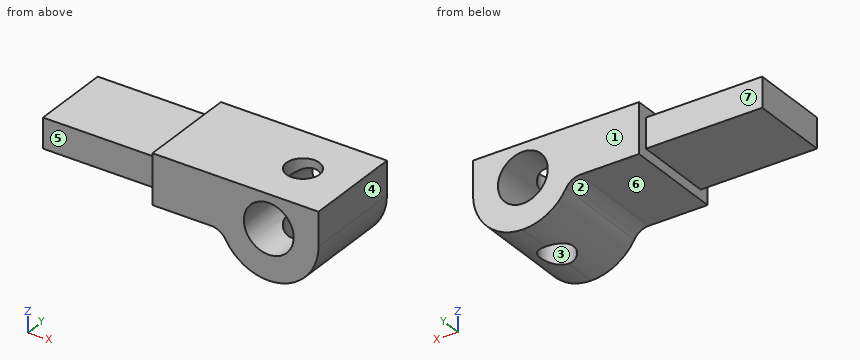
from build123d import *

# Parameters (mm, degrees)
BOSS_EXTRUDE1_DEPTH      = 38.1
BOSS_EXTRUDE1_DEPTH_BACK = 38.1
CUT_EXTRUDE1_DEPTH       = 84.279469259
CUT_EXTRUDE1_DEPTH_BACK  = 84.279469259
SKETCH4_R                = 12.7
SKETCH5_W                = 22.86
SKETCH5_H                = 60.96
BOSS_EXTRUDE2_DEPTH      = 88.9
SKETCH6_R                = 19.05
CUT_EXTRUDE2_DEPTH       = 175.596134043


with BuildPart() as part:
    # Sketch2 → Boss-Extrude1 (new, two sides: drawn at the far end of the back side and taken through both)
    with BuildSketch(Plane(origin=(0, 0, 0), x_dir=(1, 0, 0), z_dir=(0, 1, 0)).offset(-BOSS_EXTRUDE1_DEPTH_BACK)):
        with BuildLine():
            Line((-63.5, 12.7), (-63.5, -25.4))
            Line((-63.5, -25.4), (63.5, -25.4))
            Line((63.5, -25.4), (63.5, 0))
            ThreePointArc((63.5, 0), (52.340768363, 26.940768363), (25.4, 38.1))
            ThreePointArc((25.4, 38.1), (6.35, 32.995567884), (-7.595567884, 19.05))
            ThreePointArc((-7.595567884, 19.05), (-12.244090512, 14.401477372), (-18.594090512, 12.7))
            Line((-18.594090512, 12.7), (-63.5, 12.7))
        make_face()
    extrude(amount=BOSS_EXTRUDE1_DEPTH + BOSS_EXTRUDE1_DEPTH_BACK)

    # Sketch4 → Cut-Extrude1 (cut, two sides: drawn at the far end of the back side and taken through both)
    with BuildSketch(Plane.XY.offset(-CUT_EXTRUDE1_DEPTH_BACK)):
        with Locations((25.4, 0)):
            Circle(SKETCH4_R)
    extrude(amount=CUT_EXTRUDE1_DEPTH + CUT_EXTRUDE1_DEPTH_BACK, mode=Mode.SUBTRACT)

    # Sketch5 → Boss-Extrude2 (add)
    with BuildSketch(Plane.ZY.offset(63.5)):
        with Locations((6.35, 0)):
            Rectangle(SKETCH5_W, SKETCH5_H)
    extrude(amount=BOSS_EXTRUDE2_DEPTH)

    # Sketch6 → Cut-Extrude2 (cut, through all)
    with BuildSketch(Plane(origin=(0, 38.1, 0), x_dir=(1, 0, 0), z_dir=(0, 1, 0))):
        with Locations(Location((25.4, 0, 0), (0, 0, 270))):
            Circle(SKETCH6_R)
    extrude(amount=-CUT_EXTRUDE2_DEPTH, mode=Mode.SUBTRACT)


solid = part.part
Can you work these out from the model? Positions are in its coordinate system, mm. Face numbers are marked on the shaded views. A direction names the side the tool comes from. Give positions to 0.01 mm unless a question says otherwise; leave off trailing zeros. Order: outer loops, then holes, each group sorted by start corner. A loop starts at its lowest first (then second) coordinate and runs counter-clockwise, first axis right, second up. Notation, with made-up numbers: M -27,35 L 11,35 A15 ccw 11,53 Z; hole C -2.75,24.25 d4. An arc over 180 degrees is marked long. Use a Markdown table: item, result. Add a question column.
Item 1: We'd pull the mould along X, two halves only. Please class the marked faces 1, 2, 3 and 4: +X half, -X half, draft (parallel to the pull), parting line (faces both ways), or undercut.
Item 2: Suppose I cut it at D-D (y = 20). List the corners of the cut face in (x, z) for me.
Item 3: Will these pins go through, and if not, where does the flat tip stop? pin 1 (1.5 mm diameter, centred on x = -8, y = -10.5, fed in from -Z); pin 2 (8 mm diameter, centred on x = -126, y = 8, fed in from +Z); pin 3 (5 mm diameter, centred on y = -6, z = -16, fed in from +X); pin 4 (15 mm diameter, centred on x = 25.4, y = 0, fed in from +Z).
Item 4: Suppose I cut it at C-C (z = 11). List the corners of the cut face in (x, y) for me, then the cut area to 3 significant figures.
Item 5: If I drill on L1, parallel to X at y = 0, z = 20.25; L2, parallel to Z at x = 25, y = -21; L3, parallel to X at y = 21, z = 0, over which ranges is the centre line in solid material (lowest first)? Write a range as [from, to].
Item 6: Suppose I cut it at B-B (x = 42). List the corners of the cut face in (y, z) for me.
Item 7: For the marked faces 5, 6 and 7, which set-ups out of +Z, -Z, +X, -X, +Y, -Y let a thin tool reach every point of the face, with its end or its side?
Item 8: Suppose I cut it at A-A (y = 7). List the corners of the cut face in (x, z) for me.
Answer sheet:
| question | item | result |
|---|---|---|
| 1 | face 1 | draft |
| 1 | face 2 | -X half |
| 1 | face 3 | undercut |
| 1 | face 4 | +X half |
| 2 | outline | M -152.4,-5.08 L -63.5,-5.08 L -63.5,-12.7 L -18.59,-12.7 A12.7 cw -7.6,-19.05 A38.1 ccw 63.5,0 L 63.5,25.4 L -63.5,25.4 L -63.5,17.78 L -152.4,17.78 Z; hole C 25.4,0 d38.1 |
| 3 | pin 1 | stops at z = -19.64 |
| 3 | pin 2 | stops at z = 17.78 |
| 3 | pin 3 | stops at x = 61.03 |
| 3 | pin 4 | passes through |
| 4 | outline | M -152.4,-30.48 L -63.5,-30.48 L -63.5,-38.1 L 9.85,-38.1 L 9.85,38.1 L -63.5,38.1 L -63.5,30.48 L -152.4,30.48 Z; M 40.95,-38.1 L 63.5,-38.1 L 63.5,38.1 L 40.95,38.1 Z |
| 4 | area | 12,700 mm² |
| 5 | L1 | x = [-63.5, 12.7], [38.1, 63.5] |
| 5 | L2 | z = [-38.1, -19.05], [19.05, 25.4] |
| 5 | L3 | x = [-152.4, 6.35], [44.45, 63.5] |
| 6 | outline | M -38.1,-34.29 L 38.1,-34.29 L 38.1,-9.35 L -38.1,-9.35 Z; M -38.1,9.35 L 38.1,9.35 L 38.1,25.4 L -38.1,25.4 Z |
| 7 | face 5 | +Z, -Z, -X, -Y |
| 7 | face 6 | -Z, -X, +Y, -Y |
| 7 | face 7 | +Z, -Z, -X, +Y |
| 8 | outline | M -152.4,-5.08 L -63.5,-5.08 L -63.5,-12.7 L -18.59,-12.7 A12.7 cw -7.6,-19.05 A38.1 ccw 14.8,-36.6 L 14.8,-15.83 A19.05 cw 14.8,15.83 L 14.8,25.4 L -63.5,25.4 L -63.5,17.78 L -152.4,17.78 Z; M 36,-36.6 A38.1 ccw 63.5,0 L 63.5,25.4 L 36,25.4 L 36,15.83 A19.05 cw 36,-15.83 Z |
